```python
from build123d import *

# Parameters (mm, degrees)
SKETCH1_W           = 50
SKETCH1_H           = 18
BOSS_EXTRUDE2_DEPTH = 22
SKETCH4_W           = 32
SKETCH4_H           = 14
CUT_EXTRUDE1_DEPTH  = 58.515215378
SKETCH5_W           = 23
SKETCH5_H           = 18
CUT_EXTRUDE3_DEPTH  = 13
SKETCH7_W           = 50
SKETCH7_H           = 8.235017036
CUT_EXTRUDE4_DEPTH  = 58.515215378
SKETCH9_R           = 1
CUT_EXTRUDE6_DEPTH  = 54.600373133
SKETCH10_R          = 2.25
CUT_EXTRUDE7_DEPTH  = 55.895125066


with BuildPart() as part:
    # Sketch1 → Boss-Extrude2 (new body)
    with BuildSketch(Plane(origin=(0, 0, 0), x_dir=(1, 0, 0), z_dir=(0, 1, 0))):
        with Locations((25, 9)):
            Rectangle(SKETCH1_W, SKETCH1_H)
    extrude(amount=BOSS_EXTRUDE2_DEPTH)

    # Sketch4 → Cut-Extrude1 (cut, through all)
    with BuildSketch(Plane.XY):
        with Locations((25, 0)):
            Rectangle(SKETCH4_W, SKETCH4_H)
    extrude(amount=-CUT_EXTRUDE1_DEPTH, mode=Mode.SUBTRACT)

    # Sketch5 → Cut-Extrude3 (cut)
    with BuildSketch(Plane(origin=(0, 0, -18), x_dir=(-1, 0, 0), z_dir=(0, 0, -1))):
        with Locations((-25, 7)):
            Rectangle(SKETCH5_W, SKETCH5_H)
    extrude(amount=-CUT_EXTRUDE3_DEPTH, mode=Mode.SUBTRACT)

    # Sketch7 → Cut-Extrude4 (cut, through all)
    with BuildSketch(Plane(origin=(0, 0, -18), x_dir=(-1, 0, 0), z_dir=(0, 0, -1))):
        with Locations((-25, 17.882491482)):
            Rectangle(SKETCH7_W, SKETCH7_H)
    extrude(amount=-CUT_EXTRUDE4_DEPTH, mode=Mode.SUBTRACT)

    # Sketch9 → Cut-Extrude6 (cut, through all)
    with BuildSketch(Plane.XZ.offset(-7)):
        with Locations(Location((12, -11.5, 0), (0, 0, 270))):
            Circle(SKETCH9_R)
        with Locations(Location((38, -11.5, 0), (0, 0, 90))):
            Circle(SKETCH9_R)
    extrude(amount=-CUT_EXTRUDE6_DEPTH, mode=Mode.SUBTRACT)

    # Sketch10 → Cut-Extrude7 (cut, through all)
    with BuildSketch(Plane(origin=(0, 13.764982964, 0), x_dir=(1, 0, 0), z_dir=(0, 1, 0))):
        with Locations(Location((4.5, 9, 0), (0, 0, 270))):
            Circle(SKETCH10_R)
        with Locations(Location((45.5, 9, 0), (0, 0, 90))):
            Circle(SKETCH10_R)
    extrude(amount=-CUT_EXTRUDE7_DEPTH, mode=Mode.SUBTRACT)


solid = part.part
```
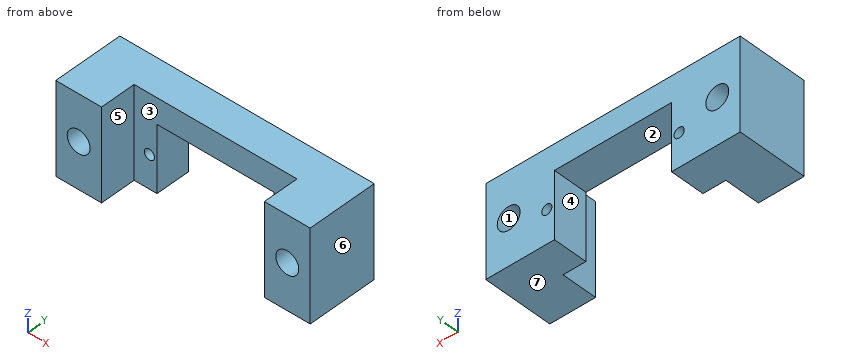
Work out the finished part from the listing and answer in its coordinate system (mm). Face numbers are marked on the shaded views. A direction names the side the tool comes from. Give positions to 0.01 mm unless a question says otherwise; leave off trailing zeros. Loops run counter-clockwise (first coordinate to the right, second up) from the corner with the lowest first, then second, coordinate; pieces in that order, holes last. Notation, with made-up numbers: (1, -27) -> (7, -27) arc R18 cw to (7, -14) -> close; hole circle Ø9 at (-9.75, 14.5). An arc over 180 degrees is marked (long way). One line per question, with ' | ' between items. Start each with the question number.
1) Determine the mould class of the marked faces 4, 5, 6 and 7 for opening direction X: +X half, -X half, draft (parallel to the pull), parting line (faces both ways), or undercut.
2) Straight lines are drawn through the part: L1, parallel to X at y = 4.75, z = -9; L2, parallel to X at y = 10.25, z = -9; L3, parallel to Z at x = 45.5, y = 8. For each, find the intervals that lie inside material, in ascending order.
3) Each of these flat-tipped pins is pushed along its axis until it touches: pin 1 (5 mm diameter, centred on x = 37.5, z = -9, fed in from -Y); pin 2 (2 mm diameter, centred on x = 24.5, y = 12, fed in from -Z). Where does it stop, or does it pass through?
4) Section B-B, the plane y = 2.75 is taken. Determine the outline of the cut face in (x, z).
5) Section D-D, the plane y = 12.25 is taken. Determine the outline of the cut face in (x, z).
6) Section A-A, the plane x = 4.5 is taken. Determine the outline of the cut face in (y, z).
7) Section C-C, the plane z = -9 is taken. Determine the outline of the cut face in (x, y), then the cut area to 3 significant figures.
8) For the marked faces 1, 2 and 3, determine the directions among +Z, -Z, +X, -X, +Y, -Y from which every point of the face is accessible in a straight line to the end or side of a thin tool.
Resolved:
1) face 4: undercut | face 5: undercut | face 6: +X half | face 7: draft
2) L1: 0 to 2.25, 6.75 to 9, 41 to 43.25, 47.75 to 50 | L2: 0 to 2.25, 6.75 to 13.5, 36.5 to 43.25, 47.75 to 50 | L3: -18 to -11.25, -6.75 to 0
3) pin 1: y = 7 | pin 2: z = -5
4) outline: (0, -18) -> (9, -18) -> (9, 0) -> (0, 0) -> close; (41, -18) -> (50, -18) -> (50, 0) -> (41, 0) -> close; hole circle Ø4.5 at (4.5, -9); hole circle Ø4.5 at (45.5, -9)
5) outline: (0, -18) -> (13.5, -18) -> (13.5, -5) -> (36.5, -5) -> (36.5, -18) -> (50, -18) -> (50, 0) -> (0, 0) -> close; hole circle Ø4.5 at (4.5, -9); hole circle Ø2 at (12, -11.5); hole circle Ø2 at (38, -11.5); hole circle Ø4.5 at (45.5, -9)
6) outline: (0, -18) -> (13.76, -18) -> (13.76, -11.25) -> (0, -11.25) -> close; (0, -6.75) -> (13.76, -6.75) -> (13.76, 0) -> (0, 0) -> close
7) outline: (0, 0) -> (2.25, 0) -> (2.25, 13.76) -> (0, 13.76) -> close; (6.75, 0) -> (9, 0) -> (9, 7) -> (13.5, 7) -> (13.5, 13.76) -> (6.75, 13.76) -> close; (36.5, 7) -> (41, 7) -> (41, 0) -> (43.25, 0) -> (43.25, 13.76) -> (36.5, 13.76) -> close; (47.75, 0) -> (50, 0) -> (50, 13.76) -> (47.75, 13.76) -> close | area: 185 mm2
8) face 1: +Y, -Y | face 2: -Z, +Y, -Y | face 3: +Z, -Z, -Y
